Autodesk Inventor part; units mm, degrees
ref_plane "YZ Plane" through (0, 0, 0) normal (1, 0, 0) x (0, 1, 0)
ref_plane "XZ Plane" through (0, 0, 0) normal (0, 1, 0) x (-1, 0, 0)
ref_plane "XY Plane" through (0, 0, 0) normal (0, 0, 1) x (1, 0, 0)
sketch "Sketch1" plane through (0, 0, 0) normal (0, 0, 1) x (1, 0, 0)
  line L0 (0, 0) -> (0, 38.1)
  line L1 (0, 38.1) -> (12.7, 38.1)
  line L2 (12.7, 38.1) -> (12.7, 12.7)
  line L3 (12.7, 12.7) -> (38.1, 12.7)
  line L4 (38.1, 12.7) -> (38.1, 0)
  line L5 (38.1, 0) -> (0, 0)
  dimension "d0" = 38.1
  dimension "d1" = 12.7
  dimension "d2" = 25.4
  dimension "d3" = 25.4
  dimension "d4" = 12.7
extrude "Extrusion1" add sketch "Sketch1" along normal blind 38.1
chamfer "Chamfer1" distance 3.175 angle 45 1 edges at (12.7, 38.1, 19.05)
chamfer "Chamfer2" distance 6.35 distance2 9.525 1 edges at (38.1, 12.7, 19.05) measured on face at (38.1, 4.2333, 12.7)
fillet "Fillet2" radius 3.175 1 edges at (12.7, 12.7, 19.05)
properties part number "Practice 6"
For this review, take the finished solid that the model builds, in its own axes (mm). A direction names the side the tool comes from. Coordinates: 2 decimals unless noted, no trailing zeros. Loops run counter-clockwise (first coordinate to the right, second up) from the corner with the lowest first, then second, coordinate; pieces in that order, holes last. Notation, with made-up numbers: (44, 37.25) -> (62, 37.25) arc R9 ccw to (62, 45.25) -> close; hole circle Ø9 at (-23, 30). An arc over 180 degrees is marked (long way). Return JSON: item names as keys, results as strings. Group by question number.
(1) For pin 1 Ø2 at (y, z) = (29.5, 24) entering from +X; pin 2 Ø14 at (x, z) = (25, 11) entering from +Y, all flat-tipped, find the tip position at first contact; note any pin that passes through.
(2) To check wall thickness, follow L1, parallel to Y at x = 20, z = 16; L2, parallel to Y at x = 14.5, z = 10.5. State the ranges of each line that lie inside material, in increasing order.
(3) Consider section C-C, the plane x = 11.5. Give the boundary of the cut face in (y, z) (3 decimals).
(4) Consider section B-B, the plane y = 21.5. Give the boundary of the cut face in (x, z), plus the area to 3 significant figures.
(5) Tool access review of faces 1 (the flat face through (12.7, 26, 19)), 2 (the flat face through (0, 19, 19)): name each direction out of +Z, -Z, +X, -X, +Y, -Y from which nothing blocks a thin tool from reaching the whole face with its end or side.
(6) Consider section A-A, the plane z = 10.5. Give the boundary of the cut face in (x, y) (3 decimals), plus the area to 3 significant figures.
Results below:
{
 "1": {"pin 1": "stops at x = 12.7", "pin 2": "stops at y = 12.7"},
 "2": {"L1": "y = 0 to 12.7", "L2": "y = 0 to 13.01"},
 "3": {"outline": "(0, 0) -> (36.125, 0) -> (36.125, 38.1) -> (0, 38.1) -> close"},
 "4": {"outline": "(0, 0) -> (12.7, 0) -> (12.7, 38.1) -> (0, 38.1) -> close", "area": "484 mm2"},
 "5": {"face 1": "+Z, -Z, +X, +Y", "face 2": "+Z, -Z, -X, +Y, -Y"},
 "6": {"outline": "(0, 0) -> (38.1, 0) -> (38.1, 6.35) -> (28.575, 12.7) -> (15.875, 12.7) arc R3.175 cw to (12.7, 15.875) -> (12.7, 34.925) -> (9.525, 38.1) -> (0, 38.1) -> close", "area": "773 mm2"}
}
